Study the drawing (mm; zero at the part's minimum x, y, z) and answer. Give positions to 0.01 mm unless a question says otherwise; leave off trailing zeros. Order: outer loops, then holes, each group sorted by start corner. A loop starts at its lowest first (then second) coordinate and runs counter-clockwise, first axis right, second up.
Item 1: Given pin 1 Ø2 at (x, y) = (694, 492) entering from -Z; pin 2 Ø25 at (y, z) = (1196.5, 517.5) entering from -X; pin 3 Ø25 at (y, z) = (1205, 356) entering from +X, each flat-ended and moving along its own axis, determine where each tip first touches the part or whether it passes through.
Item 2: A cutting plane is placed at B-B (y = 276.5). Write down the section's boundary in (x, z).
Item 3: A cutting plane is placed at A-A (z = 365). Write down the section's boundary in (x, y), plus the area to 3 significant figures.
Item 4: Find the intervals of material crossed by line 1 along Y through (x, z) = (51.5, 71.5); line 2 along Z through (x, y) = (586, 1116), in increasing order.
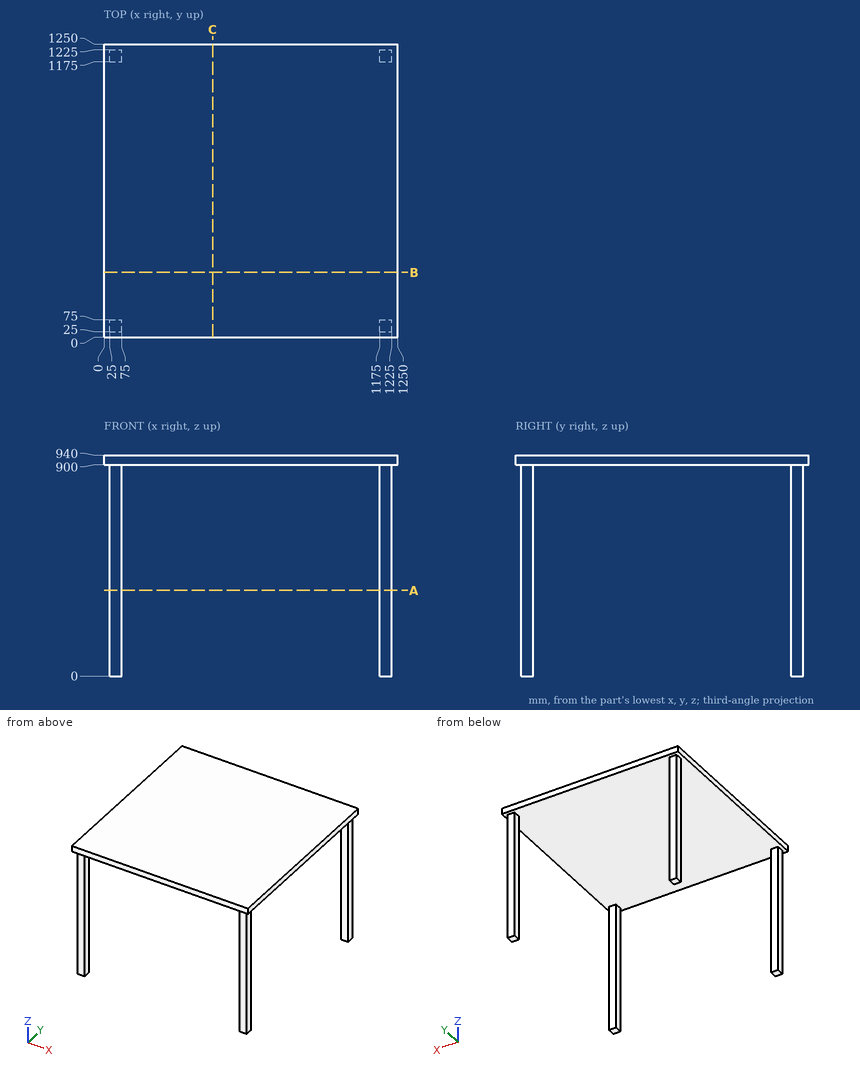
Response values:
1. pin 1: stops at z = 900
1. pin 2: stops at x = 25
1. pin 3: stops at x = 1225
2. outline: (0, 900) - (1250, 900) - (1250, 940) - (0, 940) - close
3. outline: (25, 25) - (75, 25) - (75, 75) - (25, 75) - close; (25, 1175) - (75, 1175) - (75, 1225) - (25, 1225) - close; (1175, 25) - (1225, 25) - (1225, 75) - (1175, 75) - close; (1175, 1175) - (1225, 1175) - (1225, 1225) - (1175, 1225) - close
3. area: 10,000 mm2
4. line 1: y = 25 to 75, 1175 to 1225
4. line 2: z = 900 to 940
